Source: CAD feature listing. Evaluate the final solid. Frame: model axes, mm. Round coordinates to 2 decimals unless told otherwise and drop trailing zeros. Write each loop counter-clockwise with the first axis right and the second up, starting at its lowest first coordinate (ties: lowest second). Pieces come first, ordered by that corner, then holes.
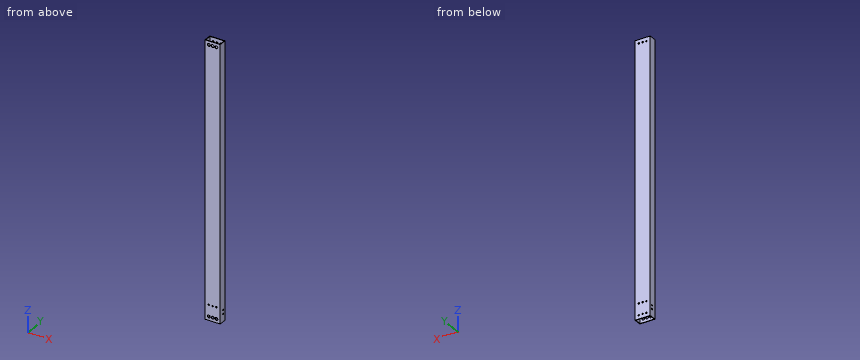
from build123d import *

# Parameters (mm, degrees)
SKETCH1_W           = 50.8
SKETCH1_H           = 25.4
SKETCH1_W_2         = 47.625
SKETCH1_H_2         = 22.225
BOSS_EXTRUDE1_DEPTH = 457.2
SKETCH3_R           = 2.5527
CUT_EXTRUDE2_DEPTH  = 1.5875
SKETCH4_R           = 4.7625
SKETCH4_R_2         = 2.5527
CUT_EXTRUDE4_DEPTH  = 1.5875
SKETCH7_R           = 2.4892
CUT_EXTRUDE5_DEPTH  = 461.188841673
SKETCH10_R          = 2.5527
CUT_EXTRUDE6_DEPTH  = 459.608940166


with BuildPart() as part:
    # Sketch1 → Boss-Extrude1 (new, symmetric)
    with BuildSketch(Plane.XY):
        Rectangle(SKETCH1_W, SKETCH1_H)
        Rectangle(SKETCH1_W_2, SKETCH1_H_2, mode=Mode.SUBTRACT)
    extrude(amount=BOSS_EXTRUDE1_DEPTH, both=True)

    # Sketch3 → Cut-Extrude2 (cut)
    with BuildSketch(Plane(origin=(0, 12.7, 0), x_dir=(1, 0, 0), z_dir=(0, 1, 0))):
        with Locations(Location((0, -444.5, 0), (0, 0, 270))):
            Circle(SKETCH3_R)
        with Locations(Location((12.7, -444.5, 0), (0, 0, 270))):
            Circle(SKETCH3_R)
        with Locations(Location((-12.7, -444.5, 0), (0, 0, 270))):
            Circle(SKETCH3_R)
        with Locations((12.7, 444.5)):
            Circle(SKETCH3_R)
        with Locations((0, 444.5)):
            Circle(SKETCH3_R)
        with Locations((-12.7, 444.5)):
            Circle(SKETCH3_R)
    extrude(amount=-CUT_EXTRUDE2_DEPTH, mode=Mode.SUBTRACT)

    # Sketch4 → Cut-Extrude4 (cut)
    with BuildSketch(Plane.XZ.offset(12.7)):
        with Locations(Location((-12.7, 444.5, 0), (0, 0, 270))):
            Circle(SKETCH4_R)
        with Locations(Location((-12.7, 444.5, 0), (0, 0, 90))):
            Circle(SKETCH4_R_2, mode=Mode.SUBTRACT)
        with Locations(Location((0, 444.5, 0), (0, 0, 270))):
            Circle(SKETCH4_R)
        with Locations(Location((0, 444.5, 0), (0, 0, 90))):
            Circle(SKETCH4_R_2, mode=Mode.SUBTRACT)
        with Locations(Location((0, 444.5, 0), (0, 0, 90))):
            Circle(SKETCH4_R_2)
        with Locations(Location((-12.7, 444.5, 0), (0, 0, 90))):
            Circle(SKETCH4_R_2)
        with Locations(Location((12.7, 444.5, 0), (0, 0, 270))):
            Circle(SKETCH4_R)
        with Locations(Location((12.7, 444.5, 0), (0, 0, 90))):
            Circle(SKETCH4_R_2, mode=Mode.SUBTRACT)
        with Locations(Location((12.7, 444.5, 0), (0, 0, 90))):
            Circle(SKETCH4_R_2)
        with Locations(Location((12.7, -444.5, 0), (0, 0, 270))):
            Circle(SKETCH4_R)
        with Locations((12.7, -444.5)):
            Circle(SKETCH4_R_2, mode=Mode.SUBTRACT)
        with Locations((12.7, -444.5)):
            Circle(SKETCH4_R_2)
        with Locations(Location((0, -444.5, 0), (0, 0, 270))):
            Circle(SKETCH4_R)
        with Locations((0, -444.5)):
            Circle(SKETCH4_R_2, mode=Mode.SUBTRACT)
        with Locations((0, -444.5)):
            Circle(SKETCH4_R_2)
        with Locations(Location((-12.7, -444.5, 0), (0, 0, 270))):
            Circle(SKETCH4_R)
        with Locations((-12.7, -444.5)):
            Circle(SKETCH4_R_2, mode=Mode.SUBTRACT)
        with Locations((-12.7, -444.5)):
            Circle(SKETCH4_R_2)
    extrude(amount=-CUT_EXTRUDE4_DEPTH, mode=Mode.SUBTRACT)

    # Sketch7 → Cut-Extrude5 (cut, through all)
    with BuildSketch(Plane(origin=(25.4, 0, 0), x_dir=(0, 0, -1), z_dir=(1, 0, 0))):
        with Locations((419.1, 3.175)):
            Circle(SKETCH7_R)
        with Locations((431.8, 3.175)):
            Circle(SKETCH7_R)
    extrude(amount=-CUT_EXTRUDE5_DEPTH, mode=Mode.SUBTRACT)

    # Sketch10 → Cut-Extrude6 (cut, through all)
    with BuildSketch(Plane(origin=(0, 12.7, 0), x_dir=(1, 0, 0), z_dir=(0, 1, 0))):
        with Locations(Location((-12.7, 406.4, 0), (0, 0, 270))):
            Circle(SKETCH10_R)
        with Locations(Location((0, 406.4, 0), (0, 0, 270))):
            Circle(SKETCH10_R)
        with Locations(Location((12.7, 406.4, 0), (0, 0, 270))):
            Circle(SKETCH10_R)
    extrude(amount=-CUT_EXTRUDE6_DEPTH, mode=Mode.SUBTRACT)


solid = part.part
1) Contact query for flat-ended pins moving along their axis: P1, Ø4.5, axis at x = 0, z = -406.4, coming from the +Y side; P2, Ø7.5, axis at x = 0, z = -444.5, coming from the -Y side. Output: stop coordinate, or through.
Taken from the geometry:
P1: passes through
P2: stops at y = 11.11
2) Section query A-A on y = -7. Return the cut outline in (x, z).
Taken from the geometry:
outline: (-25.4, -457.2) - (-23.81, -457.2) - (-23.81, 457.2) - (-25.4, 457.2) - close; (23.81, -457.2) - (25.4, -457.2) - (25.4, 457.2) - (23.81, 457.2) - close
3) Material intervals for line 1 (Z direction, x = 12, y = 11.5); line 2 (X direction, y = -11.5, z = 444.5); line 3 (Y direction, x = 8, z = 309.5), sorted ascending.
Taken from the geometry:
line 1: z = -457.2 to -446.95, -442.05 to -408.85, -403.95 to 442.05, 446.95 to 457.2
line 2: x = -25.4 to -17.46, -7.94 to -4.76, 4.76 to 7.94, 17.46 to 25.4
line 3: y = -12.7 to -11.11, 11.11 to 12.7
4) Section query B-B on z = 365. Return the cut outline in (x, y), then the cut area to 3 significant figures.
Taken from the geometry:
outline: (-25.4, -12.7) - (25.4, -12.7) - (25.4, 12.7) - (-25.4, 12.7) - close; hole (-23.81, -11.11) - (23.81, -11.11) - (23.81, 11.11) - (-23.81, 11.11) - close
area: 232 mm2
